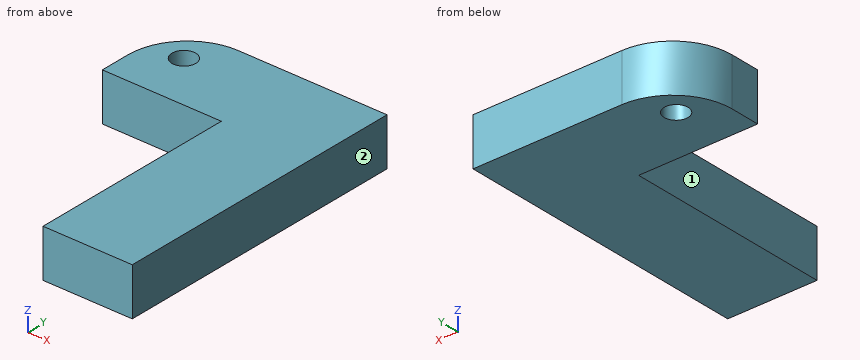
Autodesk Inventor part; units mm, degrees
ref_plane "YZ Plane" through (0, 0, 0) normal (1, 0, 0) x (0, 1, 0)
ref_plane "XZ Plane" through (0, 0, 0) normal (0, 1, 0) x (-1, 0, 0)
ref_plane "XY Plane" through (0, 0, 0) normal (0, 0, 1) x (1, 0, 0)
sketch "Sketch2" plane through (0, 0, 0) normal (0, 1, 0) x (-1, 0, 0)
  line L0 (-7.5, -4) -> (7.5, -4)
  line L1 (7.5, -4) -> (7.5, 4)
  line L2 (7.5, 4) -> (-7.5, 4)
  line L3 (-7.5, 4) -> (-7.5, -4)
  line L4 (-7.5, -4) -> (7.5, 4) construction
  line L5 (7.5, -4) -> (-7.5, 4) construction
  point P0 (0, 0)
  dimension "d5" = 15
  dimension "d6" = 8
extrude "Extrusion2" add sketch "Sketch2" along normal blind 50
sketch "Sketch3" plane through (-7.5, 0, -4) normal (-1, 0, 0) x (0, 0, 1)
  line L0 (8, 0) -> (8, 50)
  line L1 (0, 50) -> (8, 50)
  line L2 (8, 50) -> (8, 35)
  line L3 (8, 35) -> (0, 35)
  line L4 (0, 35) -> (0, 50)
  point P0 (4, 0)
  dimension "d9" = 15
extrude "Extrusion3" add sketch "Sketch3" along normal blind 20
fillet "Fillet1" radius 10 1 edges at (-27.5, 50, 0)
sketch "Sketch5" plane through (-7.5, 0, 4) normal (0, 0, 1) x (1, 0, 0)
  line L0 (-20, 35) -> (-20, 40)
  line L1 (15, 50) -> (-10, 50)
  point P0 (7.5, 0)
  point P1 (-14, 44)
  dimension "d13" = 6
  dimension "d14" = 6
hole "Hole1" at (-21.5, 44, 4) direction (0, 0, -1) diameter 4 end through all
properties part number "lever_support" material "PC/ABS Plastic"
The listing builds one solid part. Answer for the finished solid, in the listing's coordinates (mm). Face numbers are marked on the shaded views. A direction names the side the tool comes from. Coordinates: 2 decimals unless noted, no trailing zeros. Loops run counter-clockwise (first coordinate to the right, second up) from the corner with the lowest first, then second, coordinate; pieces in that order, holes last. Notation, with made-up numbers: (73.25, 60) -> (112.25, 60) arc R14 ccw to (112.25, 66) -> close; hole circle Ø2 at (64, -40). An arc over 180 degrees is marked (long way). Use one line per item in the form item = value. Start each with the question number.
Item 1: A tool of negligible diameter and unlimited length cuts with its end or side. For the marked faces 1 and 2, from which of +Z, -Z, +X, -X, +Y, -Y can it reach the whole face along a straight path? Write none if from no direction.
Item 2: The part is cut by section A-A on y = 44. Determine the outline of the cut face in (x, z).
Item 3: Consider L1, parallel to X at y = 17, z = 0.25; L2, parallel to Y at x = -21.5, z = -1.25; L3, parallel to X at y = 44, z = 1.75. Determine where each line is inside the solid, lowest interval first. Write a range as [from, to].
Item 4: The part is cut by section B-B on z = -0.25. Determine the outline of the cut face in (x, y), then the cut area to 3 significant figures.
Item 5: The part is cut by section C-C on x = -21.5. Determine the outline of the cut face in (y, z), then the cut area to 3 significant figures.
Item 6: The part is cut by section D-D on y = 7. Determine the outline of the cut face in (x, z).
Item 7: Flat-ended cylindrical pins translate along their axes: pin 1 Ø3 at (y, z) = (32, -0.5) entering from -X; pin 2 Ø2.5 at (x, z) = (-21, 1) entering from -Y. Find the tip coordinate at first contact, or state that the pin passes through.
Answer key:
q1.face_1 = +Z, -Z, -X, -Y
q1.face_2 = +Z, -Z, +X, +Y, -Y
q2.outline = (-26.67, -4) -> (-23.5, -4) -> (-23.5, 4) -> (-26.67, 4) -> close; (-19.5, -4) -> (7.5, -4) -> (7.5, 4) -> (-19.5, 4) -> close
q3.L1 = [-7.5, 7.5]
q3.L2 = [35, 42], [46, 49.17]
q3.L3 = [-26.67, -23.5], [-19.5, 7.5]
q4.outline = (-27.5, 35) -> (-7.5, 35) -> (-7.5, 0) -> (7.5, 0) -> (7.5, 50) -> (-17.5, 50) arc R10 ccw to (-27.5, 40) -> close; hole circle Ø4 at (-21.5, 44)
q4.area = 1,020 mm2
q5.outline = (35, -4) -> (42, -4) -> (42, 4) -> (35, 4) -> close; (46, -4) -> (49.17, -4) -> (49.17, 4) -> (46, 4) -> close
q5.area = 81.3 mm2
q6.outline = (-7.5, -4) -> (7.5, -4) -> (7.5, 4) -> (-7.5, 4) -> close
q7.pin_1 = -7.5
q7.pin_2 = 35
